Verification items for the finished model (mm, model axes). A direction names the side the tool comes from. Give positions to 0.01 mm unless a question says otherwise; leave off trailing zeros. Loops run counter-clockwise (first coordinate to the right, second up) from the corner with the lowest first, then second, coordinate; pieces in that order, holes last. Notation, with made-up numbers: (30, 25) -> (83, 25) arc R33 cw to (83, 58) -> close; hole circle Ø5 at (43, 24.5). An arc over 180 degrees is marked (long way). Answer in a Markdown table with one row per item. Add a question column.
Q1. Section check A-A on y = 0. Enter the section's corners in (x, z), and give its area (3 significant figures).
Q2. Section check B-B on x = 0. Enter the section's corners in (y, z).
Q3. Set-up check for faces 4 (the face through (5, 15, 2)), 5 (the face through (0, 25, 2)), 6 (the face through (-8, 5, 2)): record each of +Z, -Z, +X, -X, +Y, -Y from which the full face is reachable in a straight line by a thin tool's end or side.
Q4. Material ranges on probe 1 along Y at (x, z) = (-3.5, 3.3); probe 2 along Y at (x, z) = (-0.5, 0.65); probe 3 along Y at (x, z) = (-7.25, 3.3), recorded low to high.
Q5. Section check D-D on z = 3.25. Enter the section's corners in (x, y).
Q6. Section check C-C on x = -3. Enter the section's corners in (y, z), and give its area (3 significant figures).
Q7. Gauge pin test, flat ends, axial feed: P1, Ø1.5, axis at y = 18.5, z = 2, coming from the +X side; P2, Ø1.5, axis at x = -6, y = 20.5, coming from the -Z side. Record the tip position at first contact, or that the pin passes through.
Q8. Release check for a two-part mould opening along Y. For faces 1 (the face through (7.385, 0.751, 2.465)), 2 (the face through (7, 5, 2)), 3 (the face through (-5, 15, 2)) record: pulls with the +Y half, pulls with the -Y half, needs draft (parallel to the pull), parting line crosses it, or undercut.
```python
from build123d import *

# Parameters (mm, degrees)
SKETCH_1_W      = 20
SKETCH_1_H      = 10
SKETCH_1_R      = 2.5
EXTRUDE_1_DEPTH = 5
SKETCH_2_W      = 10
SKETCH_2_H      = 20
SKETCH_2_R      = 2
EXTRUDE_2_DEPTH = 5


with BuildPart() as part:
    # 草图1 → 凸台-拉伸1 (new body)
    with BuildSketch(Plane.XY):
        Rectangle(SKETCH_1_W, SKETCH_1_H)
        with Locations((-5, 0)):
            Circle(SKETCH_1_R, mode=Mode.SUBTRACT)
        with Locations((5, 0)):
            Circle(SKETCH_1_R, mode=Mode.SUBTRACT)
    extrude(amount=EXTRUDE_1_DEPTH)

    # 草图2 → 凸台-拉伸2 (add)
    with BuildSketch(Plane(origin=(0, 0, 0), x_dir=(-1, 0, 0), z_dir=(0, 0, -1))):
        with Locations((0, 15)):
            Rectangle(SKETCH_2_W, SKETCH_2_H)
        with Locations((0, 20)):
            Circle(SKETCH_2_R, mode=Mode.SUBTRACT)
        with Locations((0, 10)):
            Circle(SKETCH_2_R, mode=Mode.SUBTRACT)
    extrude(amount=-EXTRUDE_2_DEPTH)


solid = part.part
```
Taken from the geometry:
| question | item | result |
|---|---|---|
| 1 | outline | (-10, 0) -> (-7.5, 0) -> (-7.5, 5) -> (-10, 5) -> close; (-2.5, 0) -> (2.5, 0) -> (2.5, 5) -> (-2.5, 5) -> close; (7.5, 0) -> (10, 0) -> (10, 5) -> (7.5, 5) -> close |
| 1 | area | 50.0 mm² |
| 2 | outline | (-5, 0) -> (8, 0) -> (8, 5) -> (-5, 5) -> close; (12, 0) -> (18, 0) -> (18, 5) -> (12, 5) -> close; (22, 0) -> (25, 0) -> (25, 5) -> (22, 5) -> close |
| 3 | face 4 | +Z, -Z, +X, +Y |
| 3 | face 5 | +Z, -Z, +X, -X, +Y |
| 3 | face 6 | +Z, -Z, -X, +Y |
| 4 | probe 1 | y = -5 to -2, 2 to 25 |
| 4 | probe 2 | y = -5 to 8.06, 11.94 to 18.06, 21.94 to 25 |
| 4 | probe 3 | y = -5 to -1.09, 1.09 to 5 |
| 5 | outline | (-10, -5) -> (10, -5) -> (10, 5) -> (5, 5) -> (5, 25) -> (-5, 25) -> (-5, 5) -> (-10, 5) -> close; hole circle Ø5 at (-5, 0); hole circle Ø4 at (0, 10); hole circle Ø4 at (0, 20); hole circle Ø5 at (5, 0) |
| 6 | outline | (-5, 0) -> (-1.5, 0) -> (-1.5, 5) -> (-5, 5) -> close; (1.5, 0) -> (25, 0) -> (25, 5) -> (1.5, 5) -> close |
| 6 | area | 135 mm² |
| 7 | P1 | stops at x = 5 |
| 7 | P2 | passes through |
| 8 | face 1 | undercut |
| 8 | face 2 | pulls with the +Y half |
| 8 | face 3 | needs draft |
